```python
from build123d import *

# Parameters (mm, degrees)
SKETCH1_R           = 1.75
SKETCH1_R_2         = 1.6
SKETCH1_R_3         = 1.9
BOSS_EXTRUDE1_DEPTH = 3
FILLET1_R           = 3
FILLET2_R           = 7
FILLET3_R           = 2
SKETCH2_R           = 1.5
CUT_EXTRUDE1_DEPTH  = 10
SKETCH3_W           = 22.30502782
SKETCH3_H           = 95.515652082
CUT_EXTRUDE2_DEPTH  = 10
FILLET4_R           = 10


with BuildPart() as part:
    # Sketch1 → Boss-Extrude1 (new body)
    with BuildSketch(Plane(origin=(0, 0, 0), x_dir=(1, 0, 0), z_dir=(0, 1, 0))):
        Polygon((-75, -44), (-75, -35), (-71, -30), (-71, 30), (-75, 35), (-75, 44), (-33.772107485, 44), (-25.721646761, 41.069871925), (37.112185403, 41.069871925), (45.162646126, 44), (75, 44), (75, 26), (59.767610868, 26), (59.767610868, 30.277885673), (39.767610868, 30.277885673), (39.767610868, 26), (19, 26), (19, -26), (75, -26), (75, -44), (35.158160284, -44), (25.158160284, -34), (-11.841839716, -34), (-21.841839716, -44), align=None)
        with Locations(Location((-45, 38.5, 0), (0, 0, 270))):
            Circle(SKETCH1_R, mode=Mode.SUBTRACT)
        with Locations(Location((56, 38.5, 0), (0, 0, 270))):
            Circle(SKETCH1_R, mode=Mode.SUBTRACT)
        with Locations(Location((56, -38.5, 0), (0, 0, 270))):
            Circle(SKETCH1_R, mode=Mode.SUBTRACT)
        with Locations(Location((-45, -38.5, 0), (0, 0, 270))):
            Circle(SKETCH1_R, mode=Mode.SUBTRACT)
        with Locations(Location((23, 29, 0), (0, 0, 270))):
            Circle(SKETCH1_R_2, mode=Mode.SUBTRACT)
        with Locations(Location((72, 29, 0), (0, 0, 270))):
            Circle(SKETCH1_R_2, mode=Mode.SUBTRACT)
        with Locations(Location((72, -29, 0), (0, 0, 270))):
            Circle(SKETCH1_R_2, mode=Mode.SUBTRACT)
        with Locations(Location((23, -29, 0), (0, 0, 270))):
            Circle(SKETCH1_R_2, mode=Mode.SUBTRACT)
        with Locations(Location((-55.746480847, 37, 0), (0, 0, 270))):
            Circle(SKETCH1_R_3, mode=Mode.SUBTRACT)
        with Locations(Location((-10.235416983, 36.785886944, 0), (0, 0, 270))):
            Circle(SKETCH1_R_3, mode=Mode.SUBTRACT)
        with Locations(Location((13.764583017, 36.785886944, 0), (0, 0, 270))):
            Circle(SKETCH1_R_3, mode=Mode.SUBTRACT)
        with Locations(Location((13.764583017, -15.214113056, 0), (0, 0, 270))):
            Circle(SKETCH1_R_3, mode=Mode.SUBTRACT)
        with Locations(Location((-10.235416983, -15.214113056, 0), (0, 0, 270))):
            Circle(SKETCH1_R_3, mode=Mode.SUBTRACT)
        with Locations(Location((-55.746480847, -37, 0), (0, 0, 270))):
            Circle(SKETCH1_R_3, mode=Mode.SUBTRACT)
        with Locations(Location((-21.746480847, -37, 0), (0, 0, 270))):
            Circle(SKETCH1_R_3, mode=Mode.SUBTRACT)
        with Locations(Location((-21.746480847, 37, 0), (0, 0, 270))):
            Circle(SKETCH1_R_3, mode=Mode.SUBTRACT)
        with BuildLine():
            Line((-60, 16.45), (-60, -18.55))
            ThreePointArc((-60, -18.55), (-63.5, -22.05), (-67, -18.55))
            Line((-67, -18.55), (-67, 16.45))
            ThreePointArc((-67, 16.45), (-63.5, 19.95), (-60, 16.45))
        make_face(mode=Mode.SUBTRACT)
    extrude(amount=BOSS_EXTRUDE1_DEPTH)

    # Fillet1
    fillet1_edges = [part.edges().sort_by_distance(p)[0] for p in [
        (75, 1.5, -44),
        (75, 1.5, -26),
        (19, 1.5, -26),
        (19, 1.5, 26),
        (75, 1.5, 26),
        (75, 1.5, 44),
        (35.158160284, 1.5, 44),
        (25.158160284, 1.5, 34),
        (-11.841839716, 1.5, 34),
        (-21.841839716, 1.5, 44),
        (-75, 1.5, 44),
        (-75, 1.5, -44),
        (-33.772107485, 1.5, -44),
        (-25.721646761, 1.5, -41.069871925),
        (37.112185403, 1.5, -41.069871925),
        (45.162646126, 1.5, -44),
    ]]
    fillet(fillet1_edges, radius=FILLET1_R)

    # Fillet2
    fillet2_edges = [part.edges().sort_by_distance(p)[0] for p in [
        (-71, 1.5, 30),
        (-71, 1.5, -30),
    ]]
    fillet(fillet2_edges, radius=FILLET2_R)

    # Fillet3
    fillet3_edges = [part.edges().sort_by_distance(p)[0] for p in [
        (59.767610868, 1.5, -26),
        (59.767610868, 1.5, -30.277885673),
        (39.767610868, 1.5, -30.277885673),
        (39.767610868, 1.5, -26),
    ]]
    fillet(fillet3_edges, radius=FILLET3_R)

    # Sketch2 → Cut-Extrude1 (cut)
    with BuildSketch(Plane(origin=(0, 3, 0), x_dir=(1, 0, 0), z_dir=(0, 1, 0))):
        with Locations(Location((71, 39, 0), (0, 0, 270))):
            Circle(SKETCH2_R)
        with Locations(Location((71, -39, 0), (0, 0, 270))):
            Circle(SKETCH2_R)
    extrude(amount=-CUT_EXTRUDE1_DEPTH, mode=Mode.SUBTRACT)

    # Sketch3 → Cut-Extrude2 (cut)
    with BuildSketch(Plane(origin=(0, 3, 0), x_dir=(1, 0, 0), z_dir=(0, 1, 0))):
        with Locations((-82.15251391, 0)):
            Rectangle(SKETCH3_W, SKETCH3_H)
    extrude(amount=-CUT_EXTRUDE2_DEPTH, mode=Mode.SUBTRACT)

    # Fillet4
    fillet4_edges = [part.edges().sort_by_distance(p)[0] for p in [
        (-71, 1.5, -44),
        (-71, 1.5, 44),
    ]]
    fillet(fillet4_edges, radius=FILLET4_R)


solid = part.part
```
Can you work these out from the model? Positions are in its coordinate system, mm. A direction names the side the tool comes from. Give positions to 0.01 mm unless a question says otherwise; leave off trailing zeros. Loops run counter-clockwise (first coordinate to the right, second up) from the corner with the lowest first, then second, coordinate; pieces in that order, holes last. Notation, with made-up numbers: M 14.25,-17.5 L 27.25,-17.5 A27 ccw 27.25,16.5 Z; hole C 84,3 d6. An arc over 180 degrees is marked long. Use one line per item in the form item = value. Start each with the question number.
(1) I want a section at B-B, the plane x = 56. Write out the boundary of the cut face in (y, z).
(2) Please list where these lines run through material, in increasing order: line 1 (X direction, y = 1.6, z = 14); line 2 (X direction, y = 1.55, z = -39); line 3 (X direction, y = 1.9, z = 29).
(3) I want a section at A-A, the plane z = 7.5. Write out the boundary of the cut face in (x, y), and give its area (3 significant figures).
(4) I'm going to push flat-ended pins straight in: P1, Ø3, axis at x = -45, z = 38.5, coming from the +Y side; P2, Ø1, axis at x = -47.5, z = -18.5, coming from the -Y side; P3, Ø0.9, axis at x = 19.5, y = 1.5, coming from the -Z side; P4, Ø0.9, axis at x = 26.5, y = 1, coming from the +Z side. Where does each tip first touch, or does it pass through?
(5) I want a section at D-D, the plane y = 0.75. State how many separate pieces and enclosed holes the cut face has, and give its area (3 significant figures).
(6) Thinking about a two-plate mould opening in Z: for faces 4 (the flat face through (-60, 1, 1)), 5 (the flat face through (41.088, 1.479, -42.517)), 6 (the cylindrical face through (74.14, 1.52, -26.9)), 7 (the flat face through (7, 1, 34)), which applies, released by +Z, released by -Z, zero draft, split by the parting line, or undercut?
(7) I want a section at C-C, the plane x = -63.5. Write out the boundary of the cut face in (y, z).
(8) On a 3-axis mill with a long thin cutter (end or side, diameter ignored), from which of +Z, -Z, +X, -X, +Y, -Y can I reach the whole of each face in a straight line? I mean faces 1 (the flat face through (54, 1, 44)), 2 (the flat face through (67, 1, -26)), 3 (the flat face through (-67, 1, 1)). Say none if no direction works.
Worked out:
q1.outline = M 0,-44 L 3,-44 L 3,-40.25 L 0,-40.25 Z; M 0,-36.75 L 3,-36.75 L 3,-30.28 L 0,-30.28 Z; M 0,26 L 3,26 L 3,36.75 L 0,36.75 Z; M 0,40.25 L 3,40.25 L 3,44 L 0,44 Z
q2.line_1 = -71 to -67, -60 to -11.7, -8.77 to 12.3, 15.23 to 19
q2.line_2 = -69.66 to -46.68, -43.32 to 54.32, 57.68 to 69.5, 72.5 to 75
q2.line_3 = -71 to 21.4, 24.6 to 70.4, 73.6 to 75
q3.outline = M -71,0 L -67,0 L -67,3 L -71,3 Z; M -60,0 L 19,0 L 19,3 L -60,3 Z
q3.area = 249 mm²
q4.P1 = through
q4.P2 = 0
q4.P3 = -41.07
q4.P4 = 35.79
q5.separate_pieces = 1
q5.enclosed_holes = 19
q5.area = 8,670 mm²
q6.face_4 = undercut
q6.face_5 = released by -Z
q6.face_6 = undercut
q6.face_7 = released by +Z
q7.outline = M 0,-43.68 L 3,-43.68 L 3,-19.95 L 0,-19.95 Z; M 0,22.05 L 3,22.05 L 3,43.68 L 0,43.68 Z
q8.face_1 = +Z, +X, -X, +Y, -Y
q8.face_2 = +X, +Y, -Y
q8.face_3 = +Y, -Y
